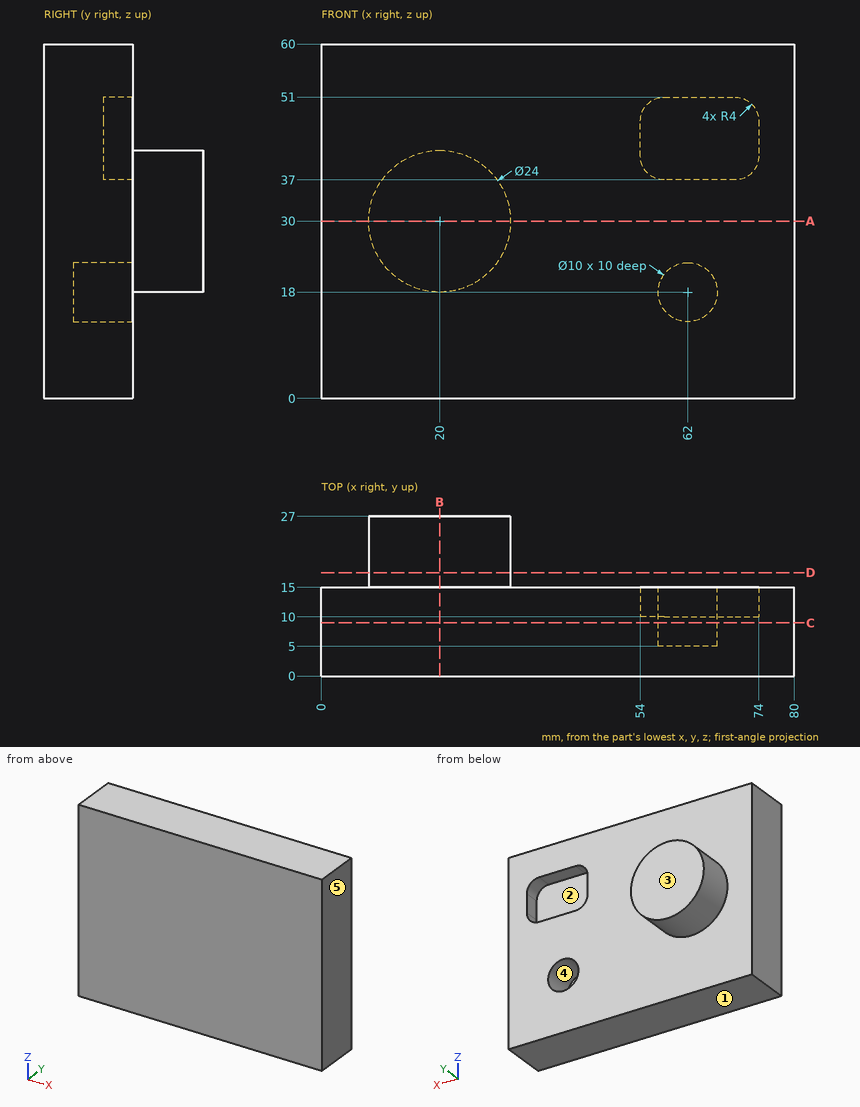
Print and shaded views of the part. All mm, measured from the part's lowest x, y and z. A direction names the side the tool comes from. Round coordinates to 2 decimals unless told otherwise and drop trailing zeros. Write each loop counter-clockwise with the first axis right and the second up, starting at its lowest first coordinate (ties: lowest second). Pieces come first, ordered by that corner, then holes.
Item 1: Cut at B-B, the plane x = 20. Give the cut face in (y, z), plus the area to 3 significant figures.
Results:
outline: (0, 0) - (15, 0) - (15, 18) - (27, 18) - (27, 42) - (15, 42) - (15, 60) - (0, 60) - close
area: 1,190 mm2
Item 2: Cut at C-C, the plane y = 9. Give the cut face in (x, z).
Results:
outline: (0, 0) - (80, 0) - (80, 60) - (0, 60) - close; hole circle Ø10 at (62, 18)
Item 3: Probe L1, parallel to X at y = 10.75, z = 18; L2, parallel to X at y = 12, z = 46; L3, parallel to Y at x = 75, z = 40. List the from-to ranges inside material, lowest first.
Results:
L1: x = 0 to 57, 67 to 80
L2: x = 0 to 54, 74 to 80
L3: y = 0 to 15
Item 4: Which spindle directions (+Z, -Z, +X, -X, +Y, -Y) get a long thin tool onto all of the face, cutting with end or side? Do the marked faces 4 and 5. Say none if no direction does.
Results:
face 4: +Y
face 5: +Z, -Z, +X, +Y, -Y
Item 5: Drop flat-ended pins along their axis: pin 1 Ø11 at (x, z) = (60, 16) entering from +Y; pin 2 Ø11 at (x, z) = (63.5, 43) entering from +Y; pin 3 Ø8 at (y, z) = (23, 44.5) entering from -X. Give the stop position or say it passes through.
Results:
pin 1: stops at y = 15
pin 2: stops at y = 10
pin 3: stops at x = 14.19
Item 6: Two-plate mould, pull along Z, no slides. Class the marked faces 1, 2 and 3: +Z half, -Z half, draft (parallel to the pull), parting line (faces both ways), or undercut.
Results:
face 1: -Z half
face 2: undercut
face 3: draft
Item 7: Cut at A-A, the plane z = 30. Give the cut face in (x, y), plus the area to 3 significant figures.
Results:
outline: (0, 0) - (80, 0) - (80, 15) - (32, 15) - (32, 27) - (8, 27) - (8, 15) - (0, 15) - close
area: 1,490 mm2
Item 8: Cut at D-D, the plane y = 17.5. Give the cut face in (x, z), plus the area to 3 significant figures.
Results:
outline: circle Ø24 at (20, 30)
area: 452 mm2
